Autodesk Inventor part; units mm, degrees
ref_plane "YZ Plane" through (0, 0, 0) normal (1, 0, 0) x (0, 1, 0)
ref_plane "XZ Plane" through (0, 0, 0) normal (0, 1, 0) x (-1, 0, 0)
ref_plane "XY Plane" through (0, 0, 0) normal (0, 0, 1) x (1, 0, 0)
sketch "草圖1" plane through (0, 0, 0) normal (0, 1, 0) x (-1, 0, 0)
  line L0 (23.5, 28.5) -> (-23.5, 28.5)
  line L1 (-28.5, 23.5) -> (-28.5, -23.5)
  line L2 (-23.5, -28.5) -> (23.5, -28.5)
  line L3 (28.5, -23.5) -> (28.5, 23.5)
  circle A0 centre (23.5, 23.5) radius 2.5
  circle A1 centre (23.5, -23.5) radius 2.5
  circle A2 centre (-23.5, -23.5) radius 2.5
  circle A3 centre (-23.5, 23.5) radius 2.5
  arc A4 (28.5, 23.5) -> (23.5, 28.5) centre (23.5, 23.5) ccw
  arc A5 (-23.5, 28.5) -> (-28.5, 23.5) centre (-23.5, 23.5) ccw
  arc A6 (-28.5, -23.5) -> (-23.5, -28.5) centre (-23.5, -23.5) ccw
  arc A7 (23.5, -28.5) -> (28.5, -23.5) centre (23.5, -23.5) ccw
  point P0 (0, 0)
  point P1 (28.5, 28.5)
  point P2 (-28.5, -28.5)
  point P3 (28.5, -28.5)
  dimension "d0" = 57
  dimension "d1" = 57
  dimension "d2" = 5
  dimension "d3" = 47
  dimension "d4" = 5
  dimension "d5" = 5
  dimension "d6" = 5
  dimension "d7" = 5
  dimension "d8" = 5
  dimension "d9" = 5
  dimension "d10" = 5
  dimension "d11" = 5
  dimension "d12" = 28.5
  dimension "d13" = 28.5
extrude "擠出1" add sketch "草圖1" along normal blind 5
sketch "草圖2" plane through (0, 5, 0) normal (0, 1, 0) x (1, 0, 0)
  circle A0 centre (0, 0) radius 19
  dimension "d16" = 38
extrude "擠出2" add sketch "草圖2" along normal blind 1.2
sketch "草圖3" plane through (0, 6.2, 0) normal (0, 1, 0) x (1, 0, 0)
  circle A0 centre (0, 0) radius 4
  dimension "d19" = 8
extrude "擠出3" add sketch "草圖3" along normal blind 20
sketch "草圖4" plane through (0, 26.2, 0) normal (0, 1, 0) x (1, 0, 0)
  line L0 (-1.8432, 3.55) -> (1.8432, 3.55)
  circle A0 centre (0, 0) radius 4
  circle A1 centre (0, 0) radius 4
  arc A2 (1.8432, 3.55) -> (-1.8432, 3.55) centre (0, 0) ccw
  line L1 (28.5, -23.5) -> (28.5, 23.5)
  point P0 (0, -4)
  dimension "d22" = 7.55
  dimension "d23" = 28.5
extrude "擠出4" cut sketch "草圖4" against normal blind 15 contours A0 L0 picked at (-0.3162, 3.662)
sketch "草圖5" plane through (0, 0, 0) normal (0, -1, 0) x (1, 0, 0)
  circle A0 centre (0, 0) radius 28.5
  dimension "d26" = 57
extrude "擠出5" add sketch "草圖5" along normal blind 9.25
sketch "草圖6" plane through (0, -9.25, 0) normal (0, -1, 0) x (1, 0, 0)
  circle A0 centre (0, 0) radius 28
  dimension "d29" = 56
extrude "擠出6" add sketch "草圖6" along normal blind 17.5
sketch "草圖7" plane through (0, -26.75, 0) normal (0, -1, 0) x (1, 0, 0)
  circle A0 centre (0, 0) radius 4
  circle A1 centre (0, 0) radius 28.5
extrude "擠出7" add sketch "草圖7" along normal blind 23 contours A0 | A1
thread "螺紋1"
properties part number "BLDC_motor"
Verification items for the finished model (mm, model axes). A direction names the side the tool comes from. Give positions to 0.01 mm unless a question says otherwise; leave off trailing zeros. Loops run counter-clockwise (first coordinate to the right, second up) from the corner with the lowest first, then second, coordinate; pieces in that order, holes last.
1. Section check A-A, the plane z = -15.5. Enter the section's corners in (x, y).
2. Section check B-B, the plane x = -11. Enter the section's corners in (y, z).
3. Thickness scan on line 1 (Z direction, x = 23.5, y = 1.6); line 2 (Y direction, x = 11.5, z = 0); line 3 (X direction, y = 2, z = -23). Record the ranges inside material, lowest first.
4. Go/stop test with flat-tipped pins: pin 1 Ø3 at (x, z) = (-10, -7.5) entering from +Y; pin 2 Ø4.5 at (x, z) = (23.5, 23.5) entering from -Y; pin 3 Ø6.5 at (x, z) = (23.5, -23.5) entering from +Y; pin 4 Ø2 at (y, z) = (-38.5, 14) entering from -X. Record where each tip stops, or that it passes through.
5. Set-up check for faces 5 (the flat face through (22, 0, -21)), 6 (the cylindrical face through (26.327, -38.089, 10.916)), 7 (the cylindrical face through (8.767, 5.592, -16.856)), 8 (the flat face through (-21.6, 0, -21.6)): record each of +Z, -Z, +X, -X, +Y, -Y from which the full face is reachable in a straight line by a thin tool's end or side.
6. Mould release check, pull along Y, two halves, no side actions. Record for faces 1 (the flat face through (-21, 0, 22)), 2 (the flat face through (0, 2, -28.5)), 3 (the flat face through (21, -9.25, -19)), 4 (the cylindrical face through (25.865, -17.877, 10.724)): released by +Y, released by -Y, zero draft, split by the parting line, or undercut.
Geometry says:
1. outline: (-28.5, 0) - (-23.92, 0) - (-23.92, -9.25) - (-23.32, -9.25) - (-23.32, -26.75) - (-23.92, -26.75) - (-23.92, -49.75) - (23.92, -49.75) - (23.92, -26.75) - (23.32, -26.75) - (23.32, -9.25) - (23.92, -9.25) - (23.92, 0) - (28.5, 0) - (28.5, 5) - (10.99, 5) - (10.99, 6.2) - (-10.99, 6.2) - (-10.99, 5) - (-28.5, 5) - close
2. outline: (-49.75, -26.29) - (-26.75, -26.29) - (-26.75, -25.75) - (-9.25, -25.75) - (-9.25, -26.29) - (0, -26.29) - (0, -28.5) - (5, -28.5) - (5, -15.49) - (6.2, -15.49) - (6.2, 15.49) - (5, 15.49) - (5, 28.5) - (0, 28.5) - (0, 26.29) - (-9.25, 26.29) - (-9.25, 25.75) - (-26.75, 25.75) - (-26.75, 26.29) - (-49.75, 26.29) - close
3. line 1: z = -28.5 to -26, -21 to 21, 26 to 28.5
3. line 2: y = -49.75 to 6.2
3. line 3: x = -28.5 to -25.95, -21.05 to 21.05, 25.95 to 28.5
4. pin 1: stops at y = 6.2
4. pin 2: passes through
4. pin 3: stops at y = 5
4. pin 4: stops at x = -25.36
5. face 5: -Z, +X, -Y
5. face 6: -Y
5. face 7: +Y
5. face 8: -Z, -X, -Y
6. face 1: released by -Y
6. face 2: zero draft
6. face 3: undercut
6. face 4: undercut
